from build123d import *

# Parameters (mm, degrees)
SKETCH003_W     = 10
SKETCH003_H     = 8
PAD002_DEPTH    = 100
SKETCH004_W     = 10
SKETCH004_H     = 3
PAD003_DEPTH    = 10
SKETCH005_R     = 1.7
POCKET001_DEPTH = 5
SKETCH006_R     = 3.5
POCKET002_DEPTH = 1
SKETCH007_W     = 10
SKETCH007_H     = 3
PAD004_DEPTH    = 10
SKETCH008_R     = 1.75
POCKET003_DEPTH = 5
SKETCH009_R     = 3.5
POCKET004_DEPTH = 1
SKETCH010_R     = 1.75
POCKET005_DEPTH = 6


with BuildPart() as part:
    # Sketch003 → Pad002 (new body)
    with BuildSketch(Plane.XY):
        with Locations((-15, 49)):
            Rectangle(SKETCH003_W, SKETCH003_H)
    extrude(amount=PAD002_DEPTH)

    # Sketch004 (on Face6 of Pad002) → Pad003 (join)
    with BuildSketch(Plane.XY.offset(100)):
        with Locations((-15, 51.5)):
            Rectangle(SKETCH004_W, SKETCH004_H)
    extrude(amount=PAD003_DEPTH)

    # Sketch005 (on Face5 of Pad003) → Pocket001 (cut)
    with BuildSketch(Plane(origin=(0, 53, 0), x_dir=(-1, 0, 0), z_dir=(0, 1, 0))):
        with Locations((15, 105)):
            Circle(SKETCH005_R)
    extrude(amount=-POCKET001_DEPTH, mode=Mode.SUBTRACT)

    # Sketch006 (on Face5 of Pocket001) → Pocket002 (cut)
    with BuildSketch(Plane(origin=(0, 53, 0), x_dir=(-1, 0, 0), z_dir=(0, 1, 0))):
        with Locations((15, 105)):
            Circle(SKETCH006_R)
    extrude(amount=-POCKET002_DEPTH, mode=Mode.SUBTRACT)

    # Sketch007 (on Face4 of Pocket002) → Pad004 (join)
    with BuildSketch(Plane(origin=(0, 0, 0), x_dir=(1, 0, 0), z_dir=(0, 0, -1))):
        with Locations((-15, -51.5)):
            Rectangle(SKETCH007_W, SKETCH007_H)
    extrude(amount=PAD004_DEPTH)

    # Sketch008 (on Face4 of Pad004) → Pocket003 (cut)
    with BuildSketch(Plane(origin=(0, 53, 0), x_dir=(-1, 0, 0), z_dir=(0, 1, 0))):
        with Locations((15, -5)):
            Circle(SKETCH008_R)
    extrude(amount=-POCKET003_DEPTH, mode=Mode.SUBTRACT)

    # Sketch009 (on Face4 of Pocket003) → Pocket004 (cut)
    with BuildSketch(Plane(origin=(0, 53, 0), x_dir=(-1, 0, 0), z_dir=(0, 1, 0))):
        with Locations((15, -5)):
            Circle(SKETCH009_R)
    extrude(amount=-POCKET004_DEPTH, mode=Mode.SUBTRACT)

    # Sketch010 (on Face6 of Pocket004) → Pocket005 (cut)
    with BuildSketch(Plane.XZ.offset(-45)):
        with Locations((-15, 90)):
            Circle(SKETCH010_R)
        with Locations((-15, 70)):
            Circle(SKETCH010_R)
        with Locations((-15, 50)):
            Circle(SKETCH010_R)
        with Locations((-15, 30)):
            Circle(SKETCH010_R)
        with Locations((-15, 10)):
            Circle(SKETCH010_R)
    extrude(amount=-POCKET005_DEPTH, mode=Mode.SUBTRACT)


solid = part.part
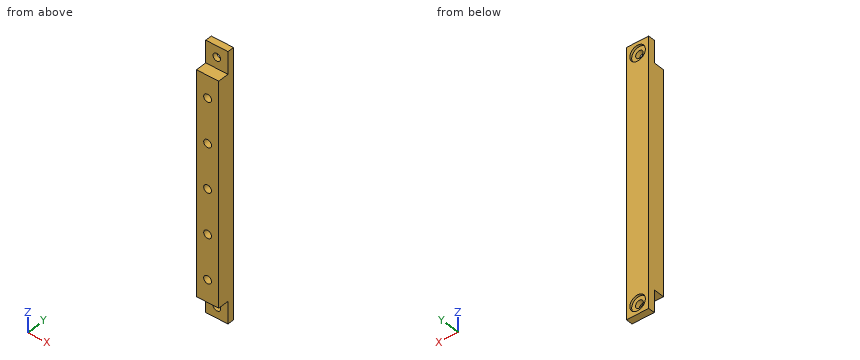
Could you check a few things on this model? Use its own coordinates, in mm. Coordinates: 2 decimals unless noted, no trailing zeros. Loops run counter-clockwise (first coordinate to the right, second up) from the corner with the lowest first, then second, coordinate; pieces in that order, holes last. Notation, with made-up numbers: (39, 61.5) -> (72, 61.5) arc R21 ccw to (72, 96.5) -> close; hole circle Ø2 at (30, 6.5). An arc over 180 degrees is marked (long way). Answer in a Markdown table with one row per item.
(1) Will these pins go through, and if not, where does the flat tip stop? pin 1 Ø2 at (x, y) = (-13.5, 48) entering from -Z; pin 2 Ø1 at (x, z) = (-15, 69.5) entering from -Y; pin 3 Ø3.5 at (x, z) = (-15, -4) entering from +Y.
Results found:
| item | result |
|---|---|
| pin 1 | stops at z = 0 |
| pin 2 | stops at y = 51 |
| pin 3 | stops at y = 52 |
(2) Imagine slicing it at B-B (y = 46.75). List the corners of the cut face in (x, z) for me.
Results found:
| item | result |
|---|---|
| outline | (-20, 0) -> (-10, 0) -> (-10, 100) -> (-20, 100) -> close; hole circle Ø3.5 at (-15, 10); hole circle Ø3.5 at (-15, 30); hole circle Ø3.5 at (-15, 50); hole circle Ø3.5 at (-15, 70); hole circle Ø3.5 at (-15, 90) |
(3) Imagine slicing it at C-C (z = 30). List the corners of the cut face in (x, y) for me.
Results found:
| item | result |
|---|---|
| outline | (-20, 45) -> (-16.75, 45) -> (-16.75, 51) -> (-13.25, 51) -> (-13.25, 45) -> (-10, 45) -> (-10, 53) -> (-20, 53) -> close |
(4) Imagine slicing it at A-A (z = 105). List the corners of the cut face in (x, y) for me, plus the area to 3 significant figures.
Results found:
| item | result |
|---|---|
| outline | (-20, 50) -> (-16.7, 50) -> (-16.7, 52) -> (-18.5, 52) -> (-18.5, 53) -> (-20, 53) -> close; (-13.3, 50) -> (-10, 50) -> (-10, 53) -> (-11.5, 53) -> (-11.5, 52) -> (-13.3, 52) -> close |
| area | 16.2 mm^2 |
(5) Imagine slicing it at D-D (z = -5). List the corners of the cut face in (x, y) for me.
Results found:
| item | result |
|---|---|
| outline | (-20, 50) -> (-16.75, 50) -> (-16.75, 52) -> (-18.5, 52) -> (-18.5, 53) -> (-20, 53) -> close; (-13.25, 50) -> (-10, 50) -> (-10, 53) -> (-11.5, 53) -> (-11.5, 52) -> (-13.25, 52) -> close |
(6) If I drill on probe 1 along Z at (x, y) = (-15, 48.55); probe 2 along Z at (x, y) = (-15, 52.75); probe 3 along X at (y, z) = (50.65, 105), over which ranges is the centre line in solid material (lowest first)?
Results found:
| item | result |
|---|---|
| probe 1 | z = 0 to 8.25, 11.75 to 28.25, 31.75 to 48.25, 51.75 to 68.25, 71.75 to 88.25, 91.75 to 100 |
| probe 2 | z = -10 to -8.5, -1.5 to 101.5, 108.5 to 110 |
| probe 3 | x = -20 to -16.7, -13.3 to -10 |
